Read the model definition and answer for the solid it produces. Units are mm, in the model's axes. A direction names the side the tool comes from. Give positions to 0.01 mm unless a question says otherwise; leave off trailing zeros. Loops run counter-clockwise (first coordinate to the right, second up) from the corner with the lowest first, then second, coordinate; pieces in that order, holes last. Notation, with made-up numbers: (75, 33.5) -> (109, 33.5) arc R14 ccw to (109, 58.5) -> close; hole circle Ø7 at (81, 21). An arc over 180 degrees is marked (long way). Return JSON: item names as keys, results as strings. Group by question number.
from build123d import *

# Parameters (mm, degrees)
SKETCH1_W           = 100
SKETCH1_H           = 100
BOSS_EXTRUDE1_DEPTH = 226
SKETCH5_W           = 35.1
SKETCH5_H           = 150
CUT_EXTRUDE1_DEPTH  = 101
BOSS_EXTRUDE2_DEPTH = 15
BOSS_EXTRUDE4_DEPTH = 19


with BuildPart() as part:
    # Sketch1 → Boss-Extrude1 (new body)
    with BuildSketch(Plane(origin=(0, 0, 0), x_dir=(1, 0, 0), z_dir=(0, 1, 0))):
        Rectangle(SKETCH1_W, SKETCH1_H)
    extrude(amount=BOSS_EXTRUDE1_DEPTH)

    # Sketch5 → Cut-Extrude1 (cut, through all)
    with BuildSketch(Plane(origin=(0, 0, -50), x_dir=(-1, 0, 0), z_dir=(0, 0, -1))):
        with Locations((-2.55, 113)):
            Rectangle(SKETCH5_W, SKETCH5_H)
    extrude(amount=-CUT_EXTRUDE1_DEPTH, mode=Mode.SUBTRACT)

    # Sketch6 → Boss-Extrude2 (add)
    with BuildSketch(Plane(origin=(-15, 0, 0), x_dir=(0, 0, -1), z_dir=(1, 0, 0))):
        with BuildLine():
            ThreePointArc((-2, 118.921359641), (-6.25, 113), (-2, 107.078640359))
            Line((-2, 107.078640359), (-2, 118.921359641))
        make_face()
        with BuildLine():
            Line((2, 118.921359641), (2, 107.078640359))
            ThreePointArc((2, 107.078640359), (6.25, 113), (2, 118.921359641))
        make_face()
        with BuildLine():
            Line((-50, 118), (-49.749371855, 118))
            ThreePointArc((-49.749371855, 118), (0, 163), (49.749371855, 118))
            Line((49.749371855, 118), (50, 118))
            Line((50, 118), (50, 188))
            Line((50, 188), (-50, 188))
            Line((-50, 188), (-50, 118))
        make_face()
        with BuildLine():
            ThreePointArc((49.749371855, 108), (0, 63), (-49.749371855, 108))
            Line((-49.749371855, 108), (-50, 108))
            Line((-50, 108), (-50, 38))
            Line((-50, 38), (50, 38))
            Line((50, 38), (50, 108))
            Line((50, 108), (49.749371855, 108))
        make_face()
    extrude(amount=BOSS_EXTRUDE2_DEPTH)

    # Sketch10 → Boss-Extrude4 (add)
    with BuildSketch(Plane.ZY.offset(-20.1)):
        with BuildLine():
            Line((-2, 119.184658438), (-2, 106.815341562))
            ThreePointArc((-2, 106.815341562), (-6.5, 113), (-2, 119.184658438))
        make_face()
        with BuildLine():
            Line((2, 119.184658438), (2, 106.815341562))
            ThreePointArc((2, 106.815341562), (6.5, 113), (2, 119.184658438))
        make_face()
    extrude(amount=BOSS_EXTRUDE4_DEPTH)


solid = part.part
1. Section A-A on z = -30 is taken. Determine the outline of the cut face in (x, y), then the cut area to 3 significant figures.
2. Straight lines are drawn through the part: line 1 (X direction, y = 120, z = 37); line 2 (Y direction, x = 17, z = -27.5); line 3 (X direction, y = 166, z = -27.5). For each, find the intervals that lie inside material, in ascending order. Write a range as from..to.
3. Section B-B on y = 172 is taken. Determine the outline of the cut face in (x, z), then the cut area to 3 significant figures.
4. Section D-D on y = 78 is taken. Determine the outline of the cut face in (x, z).
5. Which of the six approach directions +Z, -Z, +X, -X, +Y, -Y give full straight-line access (tool end or side, diameter ignored) to faces 4 (the flat face through (10, 188, -1)), 5 (the flat face through (-8, 113, 2)), 6 (the cylindrical face through (10.7, 112.9, -6.5)), 7 (the cylindrical face through (10.7, 112.9, 6.5))?
6. Determine the mould class of faces 1 (the flat face through (-50, 111, 1)), 2 (the flat face through (1.1, 113, -4)), 3 (the flat face through (-1, 226, -1)) for opening direction X: pulls with the +X half, pulls with the -X half, needs draft (parallel to the pull), parting line crosses it, or undercut.
7. Flat-ended cylindrical pins translate along their axes: pin 1 Ø6 at (x, y) = (9, 110.5) entering from -Z; pin 2 Ø3.5 at (x, y) = (15.5, 114) entering from +Z; pin 3 Ø22 at (x, z) = (7, 23.5) entering from -Y. Find the tip coordinate at first contact, or state that the pin passes through.
8. Section C-C on x = 17.5 is taken. Determine the outline of the cut face in (y, z).
Completed:
{
 "1": {"outline": "(-50, 0) -> (50, 0) -> (50, 226) -> (-50, 226) -> close; hole (-15, 73) -> (0, 73) -> (0, 38) -> (20.1, 38) -> (20.1, 188) -> (0, 188) -> (0, 153) -> (-15, 153) -> close", "area": "18,400 mm²"},
 "2": {"line 1": "x = -50..-15, 20.1..50", "line 2": "y = 0..38, 188..226", "line 3": "x = -50..0, 20.1..50"},
 "3": {"outline": "(-50, -50) -> (0, -50) -> (0, 50) -> (-50, 50) -> close; (20.1, -50) -> (50, -50) -> (50, 50) -> (20.1, 50) -> close", "area": "7,990 mm²"},
 "4": {"outline": "(-50, -50) -> (0, -50) -> (0, -35.71) -> (-15, -35.71) -> (-15, 35.71) -> (0, 35.71) -> (0, 50) -> (-50, 50) -> close; (20.1, -50) -> (50, -50) -> (50, 50) -> (20.1, 50) -> close"},
 "5": {"face 4": "+Z, -Z", "face 5": "none", "face 6": "-Z", "face 7": "+Z"},
 "6": {"face 1": "pulls with the -X half", "face 2": "undercut", "face 3": "needs draft"},
 "7": {"pin 1": "stops at z = -6.5", "pin 2": "stops at z = 6.5", "pin 3": "stops at y = 0"},
 "8": {"outline": "(0, -50) -> (38, -50) -> (38, 50) -> (0, 50) -> close; (106.82, -2) arc R6.5 ccw to (119.18, -2) -> close; (106.82, 2) -> (119.18, 2) arc R6.5 ccw to start; (188, -50) -> (226, -50) -> (226, 50) -> (188, 50) -> close"}
}
